Here's the drawing with two shaded views (mm, measured from the low corner). I have some questions. Coordinates: 2 decimals unless noted, no trailing zeros. Loops run counter-clockwise (first coordinate to the right, second up) from the corner with the lowest first, then second, coordinate; pieces in that order, holes last. Notation, with made-up numbers: (1.25, 14) -> (47.25, 14) arc R34 cw to (47.25, 49) -> close; hole circle Ø7 at (25.25, -32). An arc over 180 degrees is marked (long way). Use CSV: the item, a comma, the result in double quotes. Start each with the question number.
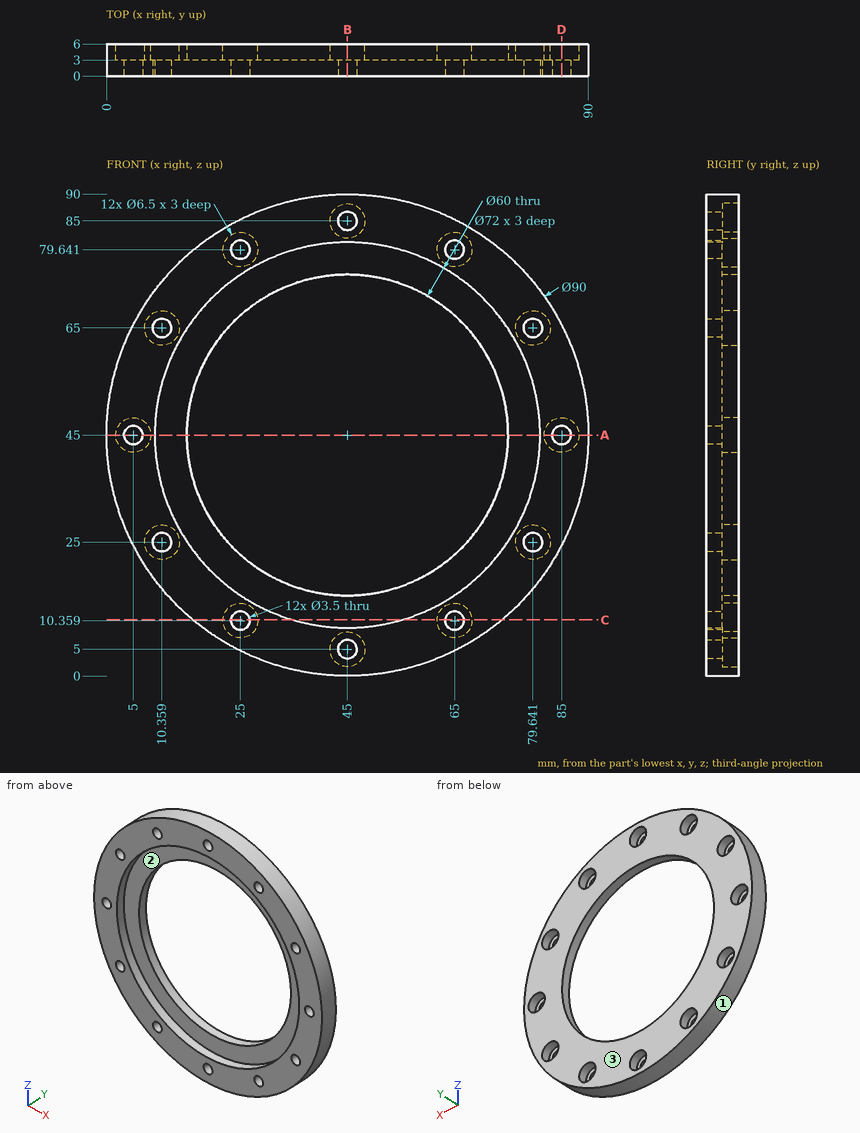
1) For P1, Ø2, axis at y = 3, z = 70, coming from the -X side; P2, Ø4.5, axis at x = 45, z = 85, coming from the +Y side; P3, Ø3, axis at x = 65, z = 79.64, coming from the +Y side; P4, Ø1, axis at x = 77, y = 1, coming from the +Z side, each with a flat end and sliding along its axis, tell me the tip position at first contact or that it passes through.
2) I want a section at C-C, the plane z = 10.5. Please give me the cut outline in (x, y).
3) Thinking about a two-plate mould opening in Z: for the marked faces 1, 2 and 3, which applies, pulls with the +Z half, pulls with the -Z half, needs draft (parallel to the pull), parting line crosses it, or undercut?
4) I want a section at A-A, the plane z = 45. Please give me the cut outline in (x, y), plus the area to 3 significant figures.
5) Please list where these lines run through material, in increasing order: L1, parallel to X at y = 4.25, z = 45; L2, parallel to X at y = 1.15, z = 65. Write a range as [from, to].
6) I want a section at D-D, the plane x = 85. Please give me the cut outline in (y, z).
7) I want a section at B-B, the plane x = 45. Please give me the cut outline in (y, z), plus the area to 3 significant figures.
Return value:
1,P1,"stops at x = 6.93"
1,P2,"stops at y = 3"
1,P3,"passes through"
1,P4,"stops at z = 77.14"
2,outline,"(16.11, 0) -> (23.26, 0) -> (23.26, 3) -> (21.75, 3) -> (21.75, 6) -> (16.11, 6) -> close; (26.74, 0) -> (34.72, 0) -> (34.72, 3) -> (55.28, 3) -> (55.28, 0) -> (63.26, 0) -> (63.26, 3) -> (61.75, 3) -> (61.75, 6) -> (28.25, 6) -> (28.25, 3) -> (26.74, 3) -> close; (66.74, 0) -> (73.89, 0) -> (73.89, 6) -> (68.25, 6) -> (68.25, 3) -> (66.74, 3) -> close"
3,face 1,"parting line crosses it"
3,face 2,"undercut"
3,face 3,"needs draft"
4,outline,"(0, 0) -> (3.25, 0) -> (3.25, 3) -> (1.75, 3) -> (1.75, 6) -> (0, 6) -> close; (6.75, 0) -> (9, 0) -> (9, 3) -> (15, 3) -> (15, 6) -> (8.25, 6) -> (8.25, 3) -> (6.75, 3) -> close; (75, 3) -> (81, 3) -> (81, 0) -> (83.25, 0) -> (83.25, 3) -> (81.75, 3) -> (81.75, 6) -> (75, 6) -> close; (86.75, 0) -> (90, 0) -> (90, 6) -> (88.25, 6) -> (88.25, 3) -> (86.75, 3) -> close"
4,area,"84.0 mm²"
5,L1,"x = [0, 1.75], [8.25, 15], [75, 81.75], [88.25, 90]"
5,L2,"x = [4.69, 8.61], [12.11, 15.07], [74.93, 77.89], [81.39, 85.31]"
6,outline,"(0, 24.38) -> (6, 24.38) -> (6, 41.75) -> (3, 41.75) -> (3, 43.25) -> (0, 43.25) -> close; (0, 46.75) -> (3, 46.75) -> (3, 48.25) -> (6, 48.25) -> (6, 65.62) -> (0, 65.62) -> close"
7,outline,"(0, 0) -> (6, 0) -> (6, 1.75) -> (3, 1.75) -> (3, 3.25) -> (0, 3.25) -> close; (0, 6.75) -> (3, 6.75) -> (3, 8.25) -> (6, 8.25) -> (6, 15) -> (3, 15) -> (3, 9) -> (0, 9) -> close; (0, 81) -> (3, 81) -> (3, 75) -> (6, 75) -> (6, 81.75) -> (3, 81.75) -> (3, 83.25) -> (0, 83.25) -> close; (0, 86.75) -> (3, 86.75) -> (3, 88.25) -> (6, 88.25) -> (6, 90) -> (0, 90) -> close"
7,area,"84.0 mm²"
